Build history of the part. All positions in model axes, mm. Face numbers are marked on the shaded views. Coordinates: 2 decimals unless noted, no trailing zeros. Order: outer loops, then holes, each group sorted by start corner. A loop starts at its lowest first (then second) coordinate and runs counter-clockwise, first axis right, second up. Notation, with made-up numbers: (27.5, 78.5) - (82.5, 78.5) arc R24 ccw to (82.5, 96.5) - close; hole circle Ø1 at (51, 10). An arc over 180 degrees is marked (long way). Answer as CSV lines item,"result". Start each with the question number.
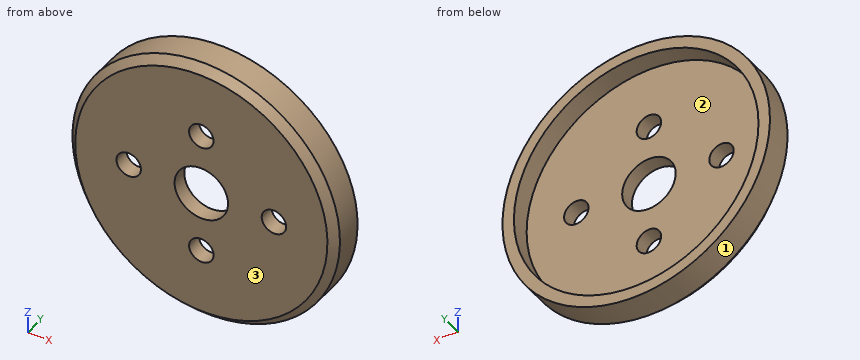
from build123d import *

# Parameters (mm, degrees)
SKETCH1_R           = 17.5
SKETCH1_R_2         = 3.5
BOSS_EXTRUDE1_DEPTH = 2
SKETCH10_R          = 17.5
SKETCH10_R_2        = 16
BOSS_EXTRUDE4_DEPTH = 2.6
SKETCH2_R           = 1.6
CUT_EXTRUDE1_DEPTH  = 3
CHAMFER2_SIZE       = 1


with BuildPart() as part:
    # Sketch1 → Boss-Extrude1 (new body)
    with BuildSketch(Plane(origin=(0, 0, 0), x_dir=(1, 0, 0), z_dir=(0, 1, 0))):
        with Locations(Location((0, 0, 0), (0, 0, 270))):
            Circle(SKETCH1_R)
        with Locations(Location((0, 0, 0), (0, 0, 270))):
            Circle(SKETCH1_R_2, mode=Mode.SUBTRACT)
    extrude(amount=BOSS_EXTRUDE1_DEPTH)

    # Sketch10 → Boss-Extrude4 (add)
    with BuildSketch(Plane(origin=(0, 2, 0), x_dir=(1, 0, 0), z_dir=(0, 1, 0))):
        with Locations(Location((0, 0, 0), (0, 0, 270))):
            Circle(SKETCH10_R)
        with Locations(Location((0, 0, 0), (0, 0, 270))):
            Circle(SKETCH10_R_2, mode=Mode.SUBTRACT)
    extrude(amount=BOSS_EXTRUDE4_DEPTH)

    # Sketch2 → Cut-Extrude1 (cut)
    with BuildSketch(Plane(origin=(0, 2, 0), x_dir=(1, 0, 0), z_dir=(0, 1, 0))):
        with Locations(Location((-9.5, 0, 0), (0, 0, 270))):
            Circle(SKETCH2_R)
        with Locations(Location((0, 8, 0), (0, 0, 270))):
            Circle(SKETCH2_R)
        with Locations(Location((0, -8, 0), (0, 0, 270))):
            Circle(SKETCH2_R)
        with Locations(Location((9.5, 0, 0), (0, 0, 270))):
            Circle(SKETCH2_R)
    extrude(amount=-CUT_EXTRUDE1_DEPTH, mode=Mode.SUBTRACT)

    # Chamfer2
    chamfer2_edges = [part.edges().sort_by_distance(p)[0] for p in [
        (0, 0, -17.5),
    ]]
    chamfer(chamfer2_edges, length=CHAMFER2_SIZE)


solid = part.part
(1) Band-saw the part on A-A on x = 0. List the corners of the cut face in (y, z).
(2) Band-saw the part on C-C on y = 3.3. List the corners of the cut face in (x, z), plus the area to 3 significant figures.
(3) Drop flat-ended pins along their axis: pin 1 Ø16 at (x, z) = (6.5, 0.5) entering from +Y; pin 2 Ø1.5 at (y, z) = (2, -2) entering from -X; pin 3 Ø1 at (x, y) = (8, 2.5) entering from -Z. Give the stop position or say it passes through.
(4) Pull direction Z, two halves, no side cores. Call the marked faces 1, 2 and 3: +Z half, -Z half, draft (parallel to the pull), parting line (faces both ways), or undercut.
(5) Probe L1, parallel to X at y = 1.25, z = 0; L2, parallel to X at y = 4.05, z = 0; L3, parallel to X at y = 0.95, z = 0. List the from-to ranges inside material, lowest first. Write a range as [from, to].
(6) Band-saw the part on B-B on z = 0. List the corners of the cut face in (x, y), plus the area to 3 significant figures.
Filled in:
1,outline,"(0, -16.5) - (1, -17.5) - (4.6, -17.5) - (4.6, -16) - (2, -16) - (2, -9.6) - (0, -9.6) - close; (0, -6.4) - (2, -6.4) - (2, -3.5) - (0, -3.5) - close; (0, 3.5) - (2, 3.5) - (2, 6.4) - (0, 6.4) - close; (0, 9.6) - (2, 9.6) - (2, 16) - (4.6, 16) - (4.6, 17.5) - (1, 17.5) - (0, 16.5) - close"
2,outline,"circle Ø35 at (0, 0); hole circle Ø32 at (0, 0)"
2,area,"158 mm^2"
3,pin 1,"stops at y = 2"
3,pin 2,"stops at x = -17.46"
3,pin 3,"stops at z = -15.81"
4,face 1,"parting line"
4,face 2,"undercut"
4,face 3,"draft"
5,L1,"x = [-17.5, -11.1], [-7.9, -3.5], [3.5, 7.9], [11.1, 17.5]"
5,L2,"x = [-17.5, -16], [16, 17.5]"
5,L3,"x = [-17.45, -11.1], [-7.9, -3.5], [3.5, 7.9], [11.1, 17.45]"
6,outline,"(-17.5, 1) - (-16.5, 0) - (-11.1, 0) - (-11.1, 2) - (-16, 2) - (-16, 4.6) - (-17.5, 4.6) - close; (-7.9, 0) - (-3.5, 0) - (-3.5, 2) - (-7.9, 2) - close; (3.5, 0) - (7.9, 0) - (7.9, 2) - (3.5, 2) - close; (11.1, 0) - (16.5, 0) - (17.5, 1) - (17.5, 4.6) - (16, 4.6) - (16, 2) - (11.1, 2) - close"
6,area,"50.0 mm^2"
